Could you check a few things on this model? Use its own coordinates, in mm. Face numbers are marked on the shaded views. A direction names the side the tool comes from. Coordinates: 2 decimals unless noted, no trailing zeros. Loops run counter-clockwise (first coordinate to the right, second up) from the corner with the lowest first, then second, coordinate; pieces in that order, holes last.
1) Imagine slicing it at D-D on x = 25. Please give me the cut outline in (y, z).
2) Imagine slicing it at C-C on y = 13.5. Please give me the cut outline in (x, z), plus the area to 3 significant figures.
3) Imagine slicing it at A-A on x = 56.5. Please give me the cut outline in (y, z), plus the area to 3 significant figures.
4) Thinking about a two-plate mould opening in Y: for the marked faces 3, 4 and 5, which applies, released by +Y, released by -Y, zero draft, split by the parting line, or undercut?
5) If I drill on line 1 along X through (y, z) = (32, 17.5); line 2 along X through (y, z) = (9, -13.5); line 3 along Z through (x, y) = (72, 23), over which ranges is the centre line in solid material (lowest first)?
6) Will these pins go through, and if not, where does the flat tip stop? P1, Ø3.5, axis at x = 82.5, z = -2.5, coming from the -Y side; P2, Ø4, axis at y = 18, z = 16, coming from the -X side; P3, Ø12, axis at x = -75.5, y = 14, coming from the +Z side; P4, Ø6, axis at x = 100.26, z = -0.02, coming from the -Y side.
7) For the marked faces 1 and 2, which set-ups out of +Z, -Z, +X, -X, +Y, -Y let a thin tool reach every point of the face, with its end or its side?
8) Imagine slicing it at B-B on y = 28. Please give me the cut outline in (x, z).
```python
from build123d import *

# Parameters (mm, degrees)
SKETCH1_W           = 203.2
SKETCH1_H           = 38.1
BOSS_EXTRUDE1_DEPTH = 39.69258
SKETCH3_R           = 1.905
CUT_EXTRUDE1_DEPTH  = 40.69258
SKETCH4_R           = 3.3782
CUT_EXTRUDE3_DEPTH  = 40.69258
CUT_EXTRUDE5_DEPTH  = 6.35
SKETCH7_W           = 7.62
SKETCH7_H           = 38.1
CUT_EXTRUDE6_DEPTH  = 29.21
SKETCH8_W           = 152.4
SKETCH8_H           = 19.05
BOSS_EXTRUDE2_DEPTH = 3.175
SKETCH9_R           = 1.778
CUT_EXTRUDE7_DEPTH  = 3.175
SKETCH10_W          = 20.32
SKETCH10_H          = 12.7
CUT_EXTRUDE8_DEPTH  = 38.1
SCALE1_SCALE        = 1.02


with BuildPart() as part:
    # Sketch1 → Boss-Extrude1 (new body)
    with BuildSketch(Plane(origin=(0, 0, 0), x_dir=(1, 0, 0), z_dir=(0, 1, 0))):
        Rectangle(SKETCH1_W, SKETCH1_H)
    extrude(amount=BOSS_EXTRUDE1_DEPTH)

    # Sketch3 → Cut-Extrude1 (cut, through all)
    with BuildSketch(Plane.XZ):
        with Locations((-98.298, 14.732)):
            Circle(SKETCH3_R)
        with Locations((-98.298, 0)):
            Circle(SKETCH3_R)
        with Locations((-98.298, -14.732)):
            Circle(SKETCH3_R)
    cut_extrude1 = extrude(amount=-CUT_EXTRUDE1_DEPTH, mode=Mode.SUBTRACT)

    # Mirror1: Cut-Extrude1 across plane
    add(cut_extrude1.mirror(Plane(origin=(0, 0, 0), x_dir=(0, 0, 1), z_dir=(1, 0, 0))), mode=Mode.SUBTRACT)

    # Sketch4 → Cut-Extrude3 (cut, through all)
    with BuildSketch(Plane(origin=(0, 39.69258, 0), x_dir=(1, 0, 0), z_dir=(0, 1, 0))):
        Circle(SKETCH4_R)
        with Locations((81.28, 0)):
            Circle(SKETCH4_R)
        with Locations((-81.28, 0)):
            Circle(SKETCH4_R)
    extrude(amount=-CUT_EXTRUDE3_DEPTH, mode=Mode.SUBTRACT)

    # Sketch6 → Cut-Extrude5 (cut)
    with BuildSketch(Plane.XZ):
        Polygon((86.995, 3.299556788), (81.28, 6.599113577), (75.565, 3.299556788), (75.565, -3.299556788), (81.28, -6.599113577), (86.995, -3.299556788), align=None)
        Polygon((-86.995, -3.299556788), (-86.995, 3.299556788), (-81.28, 6.599113577), (-75.565, 3.299556788), (-75.565, -3.299556788), (-81.28, -6.599113577), align=None)
        Polygon((5.715, 3.299556788), (0, 6.599113577), (-5.715, 3.299556788), (-5.715, -3.299556788), (0, -6.599113577), (5.715, -3.299556788), align=None)
    extrude(amount=-CUT_EXTRUDE5_DEPTH, mode=Mode.SUBTRACT)

    # Sketch7 → Cut-Extrude6 (cut)
    with BuildSketch(Plane(origin=(0, 39.69258, 0), x_dir=(1, 0, 0), z_dir=(0, 1, 0))):
        with Locations((-97.79, 0)):
            Rectangle(SKETCH7_W, SKETCH7_H)
        with Locations((97.79, 0)):
            Rectangle(SKETCH7_W, SKETCH7_H)
    extrude(amount=-CUT_EXTRUDE6_DEPTH, mode=Mode.SUBTRACT)

    # Sketch8 → Boss-Extrude2 (add)
    with BuildSketch(Plane(origin=(0, 39.69258, 0), x_dir=(1, 0, 0), z_dir=(0, 1, 0))):
        with Locations((0, -28.575)):
            Rectangle(SKETCH8_W, SKETCH8_H)
    extrude(amount=-BOSS_EXTRUDE2_DEPTH)

    # Sketch9 → Cut-Extrude7 (cut)
    with BuildSketch(Plane.XZ.offset(-36.51758)):
        with Locations((29.21, 31.75)):
            Circle(SKETCH9_R)
        with Locations((66.21018, 31.75)):
            Circle(SKETCH9_R)
    cut_extrude7 = extrude(amount=-CUT_EXTRUDE7_DEPTH, mode=Mode.SUBTRACT)

    # Mirror2: Cut-Extrude7 across plane
    add(cut_extrude7.mirror(Plane(origin=(0, 0, 0), x_dir=(0, 0, 1), z_dir=(1, 0, 0))), mode=Mode.SUBTRACT)

    # Sketch10 → Cut-Extrude8 (cut)
    with BuildSketch(Plane.XY.offset(19.05)):
        with Locations((48.26, 30.16758)):
            Rectangle(SKETCH10_W, SKETCH10_H)
    cut_extrude8 = extrude(amount=-CUT_EXTRUDE8_DEPTH, mode=Mode.SUBTRACT)

    # Mirror3: Cut-Extrude8 across plane
    add(cut_extrude8.mirror(Plane(origin=(0, 0, 0), x_dir=(0, 0, 1), z_dir=(1, 0, 0))), mode=Mode.SUBTRACT)


with BuildPart() as part_1:
    # Scale1: scaled about (0, 19.51392143, 0.949094237)
    add(part.part.scale(SCALE1_SCALE).moved(Location((0, -0.390278429, -0.018981885))))


solid = part_1.part
```
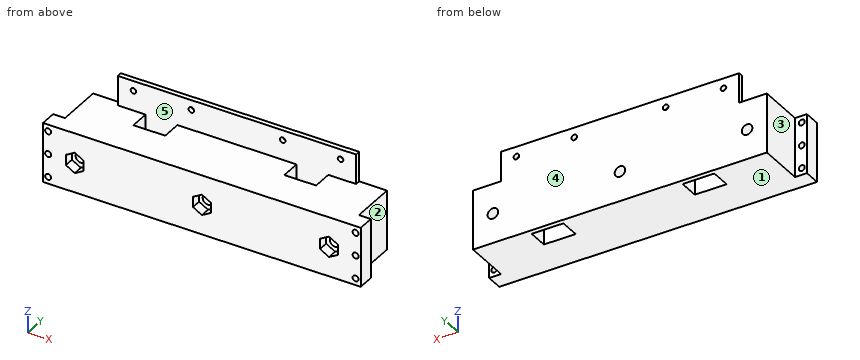
Filled in:
1. outline: (-0.39, -19.45) - (40.1, -19.45) - (40.1, 38.84) - (36.86, 38.84) - (36.86, 19.41) - (-0.39, 19.41) - close
2. outline: (-95.86, -19.45) - (95.86, -19.45) - (95.86, 19.41) - (-95.86, 19.41) - close; hole circle Ø6.89 at (-82.91, -0.02); hole circle Ø6.89 at (0, -0.02); hole circle Ø6.89 at (82.91, -0.02)
2. area: 7,340 mm2
3. outline: (-0.39, -19.45) - (23.9, -19.45) - (23.9, 19.41) - (-0.39, 19.41) - close; (36.86, -19.45) - (40.1, -19.45) - (40.1, 38.84) - (36.86, 38.84) - close
3. area: 1,130 mm2
4. face 3: zero draft
4. face 4: released by +Y
4. face 5: undercut
5. line 1: x = -95.86 to -59.59, -38.86 to 38.86, 59.59 to 95.86
5. line 2: x = -103.63 to -101.44, -99.09 to 99.09, 101.44 to 103.63
5. line 3: z = -19.45 to 19.41
6. P1: stops at y = 6.09
6. P2: stops at x = -95.86
6. P3: stops at z = 19.41
6. P4: stops at y = -0.39
7. face 1: -Z, +X, -X, +Y, -Y
7. face 2: +Z, -Z, +X, +Y
8. outline: (-95.86, -19.45) - (-59.59, -19.45) - (-59.59, 19.41) - (-95.86, 19.41) - close; (-38.86, -19.45) - (38.86, -19.45) - (38.86, 19.41) - (-38.86, 19.41) - close; (59.59, -19.45) - (95.86, -19.45) - (95.86, 19.41) - (59.59, 19.41) - close; hole circle Ø6.89 at (-82.91, -0.02); hole circle Ø6.89 at (0, -0.02); hole circle Ø6.89 at (82.91, -0.02)
